```python
from build123d import *

# Parameters (mm, degrees)
ESQUISSE1_W                  = 8
ESQUISSE1_H                  = 10
BOSS_EXTRU_1_DEPTH           = 28
ESQUISSE2_R                  = 2.25
ENL_V_MAT_EXTRU_1_DEPTH      = 11
ESQUISSE3_R                  = 3.15
ENL_V_MAT_EXTRU_2_DEPTH      = 1
ENL_V_MAT_EXTRU_2_DEPTH_BACK = 9
ESQUISSE4_R                  = 3.65
ENL_V_MAT_EXTRU_3_DEPTH      = 1


with BuildPart() as part:
    # Esquisse1 → Boss.-Extru.1 (new body)
    with BuildSketch(Plane.XY):
        with Locations((4, 5)):
            Rectangle(ESQUISSE1_W, ESQUISSE1_H)
    extrude(amount=BOSS_EXTRU_1_DEPTH)

    # Esquisse2 → Enlèv. mat.-Extru.1 (cut, through all)
    with BuildSketch(Plane(origin=(0, 10, 0), x_dir=(1, 0, 0), z_dir=(0, 1, 0))):
        with Locations((4, -24)):
            Circle(ESQUISSE2_R)
        with Locations((4, -4)):
            Circle(ESQUISSE2_R)
    extrude(amount=-ENL_V_MAT_EXTRU_1_DEPTH, mode=Mode.SUBTRACT)

    # Esquisse3 → Enlèv. mat.-Extru.2 (cut, two sides)
    with BuildSketch(Plane.ZY) as enl_v_mat_extru_2_sk:
        with Locations((14, 5)):
            Circle(ESQUISSE3_R)
    extrude(amount=ENL_V_MAT_EXTRU_2_DEPTH, mode=Mode.SUBTRACT)
    extrude(enl_v_mat_extru_2_sk.sketch, amount=-ENL_V_MAT_EXTRU_2_DEPTH_BACK, mode=Mode.SUBTRACT)

    # Esquisse4 → Enlèv. mat.-Extru.3 (cut)
    with BuildSketch(Plane.ZY):
        with Locations((14, 5)):
            Circle(ESQUISSE4_R)
    extrude(amount=-ENL_V_MAT_EXTRU_3_DEPTH, mode=Mode.SUBTRACT)


solid = part.part
```
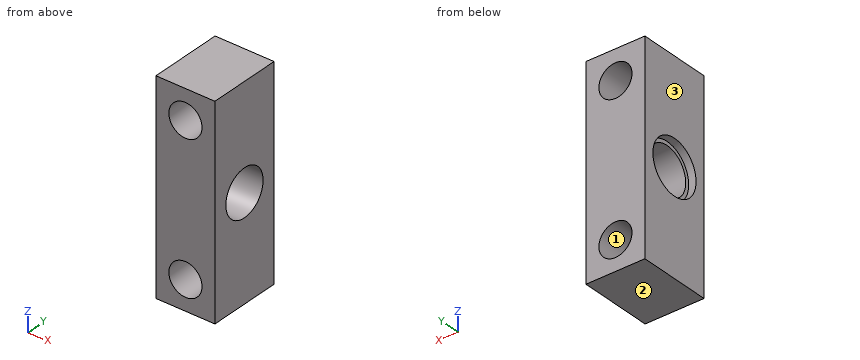
Check sheet for the modelled part. Datum: model origin and axes. Units: mm. Face numbers are marked on the shaded views. Give positions to 0.01 mm unless a question says otherwise; leave off trailing zeros. Write each loop counter-clockwise with the first axis right and the second up, starting at its lowest first coordinate (ties: lowest second). Pieces come first, ordered by that corner, then holes. Notation, with made-up numbers: (70.5, -8) - (101.5, -8) arc R22 cw to (101.5, 21) - close; hole circle Ø9 at (-10, 18). An arc over 180 degrees is marked (long way). Answer as a JSON object with one key per item and string values. Group by question number.
1) Release check for a two-part mould opening along Z. For the marked faces 1, 2 and 3 record: pulls with the +Z half, pulls with the -Z half, needs draft (parallel to the pull), parting line crosses it, or undercut.
2) Thickness scan on probe 1 along X at (y, z) = (7.5, 24); probe 2 along Z at (x, y) = (5, 8.75); probe 3 along Z at (x, y) = (5.5, 3.75). Record the ranges inside material, lowest first. Write a range as from..to.
3) Sectioned sample at A-A (x = 4). Record the cut outline in (y, z), then the cut area to 3 significant figures.
4) Sectioned sample at D-D (x = 7). Record the cut outline in (y, z).
5) Depth check by flat-ended pin: P1, Ø1.5, axis at x = 3.5, y = 5, coming from the -Z side. Enter the tip coordinate at first touch or a pass-through.
6) Sectioned sample at C-C (y = 2.25). Record the cut outline in (x, z).
7) Sectioned sample at B-B (z = 14). Record the cut outline in (x, y).
Geometry results:
{
 "1": {"face 1": "undercut", "face 2": "pulls with the -Z half", "face 3": "needs draft"},
 "2": {"probe 1": "x = 0..1.75, 6.25..8", "probe 2": "z = 0..1.98, 6.02..21.98, 26.02..28", "probe 3": "z = 0..2.32, 5.68..11.11, 16.89..22.32, 25.68..28"},
 "3": {"outline": "(0, 0) - (10, 0) - (10, 1.75) - (0, 1.75) - close; (0, 6.25) - (10, 6.25) - (10, 21.75) - (0, 21.75) - close; (0, 26.25) - (10, 26.25) - (10, 28) - (0, 28) - close; hole circle Ø6.3 at (5, 14)", "area": "159 mm^2"},
 "4": {"outline": "(0, 0) - (10, 0) - (10, 28) - (0, 28) - close; hole circle Ø6.3 at (5, 14)"},
 "5": {"P1": "stops at z = 0"},
 "6": {"outline": "(0, 0) - (8, 0) - (8, 12.46) - (1, 12.46) - (1, 11.6) - (0, 11.6) - close; (0, 16.4) - (1, 16.4) - (1, 15.54) - (8, 15.54) - (8, 28) - (0, 28) - close; hole circle Ø4.5 at (4, 4); hole circle Ø4.5 at (4, 24)"},
 "7": {"outline": "(0, 0) - (8, 0) - (8, 1.85) - (1, 1.85) - (1, 1.35) - (0, 1.35) - close; (0, 8.65) - (1, 8.65) - (1, 8.15) - (8, 8.15) - (8, 10) - (0, 10) - close"}
}
